```python
from build123d import *

# Parameters (mm, degrees)
BOSS_EXTRUDE1_DEPTH = 10
SKETCH2_R           = 3.5
SKETCH2_R_2         = 1.75
CUT_EXTRUDE1_DEPTH  = 1.55
SKETCH2_2_R         = 1.75
CUT_EXTRUDE2_DEPTH  = 6.6


with BuildPart() as part:
    # Sketch1 → Boss-Extrude1 (new body)
    with BuildSketch(Plane(origin=(0, 0, 0), x_dir=(0, 0, -1), z_dir=(1, 0, 0))):
        Polygon((-32, 5.5), (-32, -0.5), (32, -0.5), (32, 5.5), (27, 5.5), (27, 0.5), (-27, 0.5), (-27, 5.5), align=None)
    extrude(amount=BOSS_EXTRUDE1_DEPTH)

    # Sketch2 → Cut-Extrude1 (cut, symmetric)
    with BuildSketch(Plane.XY.offset(29.5)):
        with Locations((5, 5.5)):
            Circle(SKETCH2_R)
        with Locations((5, 5.5)):
            Circle(SKETCH2_R_2, mode=Mode.SUBTRACT)
    cut_extrude1 = extrude(amount=CUT_EXTRUDE1_DEPTH, both=True, mode=Mode.SUBTRACT)

    # Sketch2<2> → Cut-Extrude2 (cut, symmetric)
    with BuildSketch(Plane.XY.offset(29.5)):
        with Locations((5, 5.5)):
            Circle(SKETCH2_2_R)
    cut_extrude2 = extrude(amount=CUT_EXTRUDE2_DEPTH, both=True, mode=Mode.SUBTRACT)

    # Mirror1: Cut-Extrude1 across plane
    add(cut_extrude1.mirror(Plane.XY), mode=Mode.SUBTRACT)

    # Mirror2: Cut-Extrude2 across plane
    add(cut_extrude2.mirror(Plane.XY), mode=Mode.SUBTRACT)


solid = part.part
```
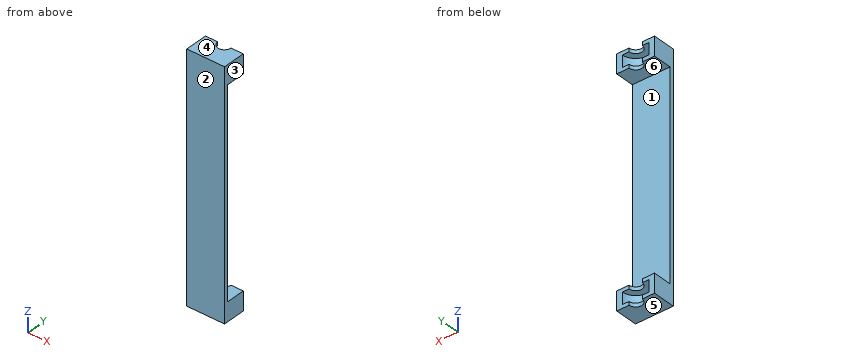
Geometry check sheet. Reference: the model listing, model coordinates, mm. Face numbers are marked on the shaded views. A direction names the side the tool comes from. Coordinates: 2 decimals unless noted, no trailing zeros. Loops run counter-clockwise (first coordinate to the right, second up) from the corner with the lowest first, then second, coordinate; pieces in that order, holes last.
Item 1: Go/stop test with flat-tipped pins: pin 1 Ø5 at (x, z) = (2.5, 9) entering from +Y; pin 2 Ø1.8 at (x, y) = (6, 4.5) entering from -Z. Record where each tip stops, or that it passes through.
Item 2: Release check for a two-part mould opening along Z. For the marked faces 3, 4, 5 and 6 record: released by +Z, released by -Z, zero draft, split by the parting line, or undercut.
Item 3: Sectioned sample at C-C, the plane z = 16.5. Record the boundary of the cut face in (x, y), then the cut area to 3 significant figures.
Item 4: Sectioned sample at B-B, the plane x = 5. Record the boundary of the cut face in (y, z).
Item 5: Thickness scan on line 1 (Z direction, x = 3.5, y = 3.3); line 2 (Z direction, x = 5.5, y = 1); line 3 (Y direction, x = 2.75, z = -2.5). Record the ranges inside material, lowest first.
Item 6: Sectioned sample at A-A, the plane y = 3.05. Record the boundary of the cut face in (x, z).
Item 7: Access from +Z, -Z, +X, -X, +Y, -Y to the whole of each face (thin tool, end or side, straight path). Record for the marked faces 1 and 2.
Check result:
1. pin 1: stops at y = 0.5
1. pin 2: stops at z = -32
2. face 3: zero draft
2. face 4: released by +Z
2. face 5: released by -Z
2. face 6: undercut
3. outline: (0, -0.5) - (10, -0.5) - (10, 0.5) - (0, 0.5) - close
3. area: 10.0 mm2
4. outline: (-0.5, -32) - (3.75, -32) - (3.75, -31.05) - (2, -31.05) - (2, -27.95) - (3.75, -27.95) - (3.75, -27) - (0.5, -27) - (0.5, 27) - (3.75, 27) - (3.75, 27.95) - (2, 27.95) - (2, 31.05) - (3.75, 31.05) - (3.75, 32) - (-0.5, 32) - close
5. line 1: z = -32 to -31.05, -27.95 to -27, 27 to 27.95, 31.05 to 32
5. line 2: z = -32 to -27, 27 to 32
5. line 3: y = -0.5 to 0.5
6. outline: (0, -32) - (10, -32) - (10, -27) - (0, -27) - close; (0, 27) - (10, 27) - (10, 32) - (0, 32) - close; hole (2.5, -31.05) - (7.5, -31.05) - (7.5, -27.95) - (2.5, -27.95) - close; hole (2.5, 27.95) - (7.5, 27.95) - (7.5, 31.05) - (2.5, 31.05) - close
7. face 1: +X, -X, +Y
7. face 2: +Z, -Z, +X, -X, -Y
